Part model, mm, in its own coordinate system. Give positions to 0.01 mm unless a question says otherwise; leave off trailing zeros. Order: outer loops, then holes, each group sorted by start corner. A loop starts at its lowest first (then second) coordinate and runs counter-clockwise, first axis right, second up. Notation, with made-up numbers: M 70,58 L 123,58 A13 cw 123,66 Z; hole C 16.25,61.5 d10. An arc over 180 degrees is marked long. Answer as a JSON object with one key per item and string values.
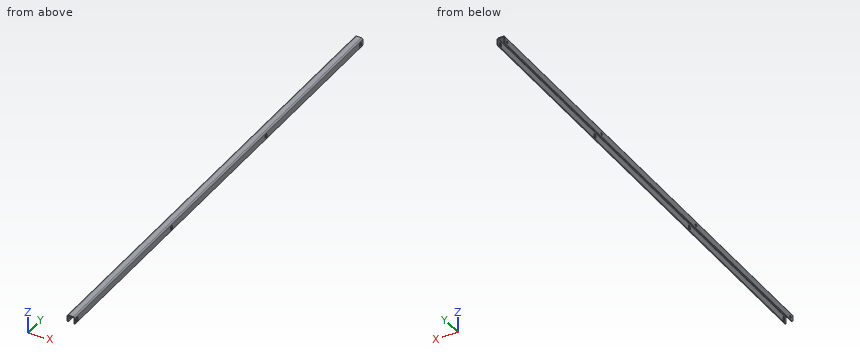
from build123d import *

# Parameters (mm, degrees)
BASE_FLANGE1_DEPTH = 1613
CUT_EXTRUDE1_REACH = 1615.344
SKETCH6_R          = 4.5
FILLET1_R          = 3
CUT_EXTRUDE2_REACH = 1615.344
LPATTERN1_COUNT    = 4
LPATTERN1_PITCH    = 529


# Sheet-metal steps are written as plain solids
with BuildPart() as part:
    # Sketch1 → Base-Flange1 (new body)
    with BuildSketch(Plane(origin=(0, 0, 0), x_dir=(1, 0, 0), z_dir=(0, 1, 0))):
        with BuildLine():
            Line((-12.5, 25), (-12.5, 4.5))
            ThreePointArc((-12.5, 4.5), (-11.181980515, 1.318019485), (-8, 0))
            Line((-8, 0), (8, 0))
            ThreePointArc((8, 0), (11.181980515, 1.318019485), (12.5, 4.5))
            Line((12.5, 4.5), (12.5, 25))
            Line((12.5, 25), (9.5, 25))
            Line((9.5, 25), (9.5, 4.5))
            ThreePointArc((9.5, 4.5), (9.060660172, 3.439339828), (8, 3))
            Line((8, 3), (-8, 3))
            ThreePointArc((-8, 3), (-9.060660172, 3.439339828), (-9.5, 4.5))
            Line((-9.5, 4.5), (-9.5, 25))
            Line((-9.5, 25), (-12.5, 25))
        make_face()
    extrude(amount=BASE_FLANGE1_DEPTH)

    # Sketch6 → Cut-Extrude1 (cut, up to next)
    with BuildSketch(Plane(origin=(-9.5, 0, 0), x_dir=(0, 0, -1), z_dir=(1, 0, 0)), mode=Mode.PRIVATE) as cut_extrude1_sk1:
        with Locations((15.5, 13)):
            Circle(SKETCH6_R)
    cut_extrude1_tool1 = extrude(cut_extrude1_sk1.sketch, amount=-CUT_EXTRUDE1_REACH, mode=Mode.PRIVATE) & part.part
    cut_extrude1 = cut_extrude1_tool1.solids().sort_by_distance((-9.5, 13, -15.5))[0]
    add(cut_extrude1, mode=Mode.SUBTRACT)

    # Fillet1
    fillet1_edges = [part.edges().sort_by_distance(p)[0] for p in [
        (11, 0, -25),
        (-11, 0, -25),
        (11, 1613, -25),
        (-11, 1613, -25),
    ]]
    fillet(fillet1_edges, radius=FILLET1_R)

    # Sketch7 → Cut-Extrude2 (cut, up to next)
    with BuildSketch(Plane.ZY.offset(-9.5), mode=Mode.PRIVATE) as cut_extrude2_sk1:
        with BuildLine():
            Line((-18.5, 18), (-12.5, 18))
            ThreePointArc((-12.5, 18), (-7.5, 13), (-12.5, 8))
            Line((-12.5, 8), (-18.5, 8))
            ThreePointArc((-18.5, 8), (-23.5, 13), (-18.5, 18))
        make_face()
    cut_extrude2_tool1 = extrude(cut_extrude2_sk1.sketch, amount=-CUT_EXTRUDE2_REACH, mode=Mode.PRIVATE) & part.part
    cut_extrude2 = cut_extrude2_tool1.solids().sort_by_distance((9.5, 13, -15.5))[0]
    add(cut_extrude2, mode=Mode.SUBTRACT)

    # LPattern1: Cut-Extrude1, Cut-Extrude2 ×4
    with Locations(*[(0, i * LPATTERN1_PITCH, 0) for i in range(1, LPATTERN1_COUNT)]):
        add(cut_extrude1, mode=Mode.SUBTRACT)
        add(cut_extrude2, mode=Mode.SUBTRACT)


solid = part.part
1. Pin check, flat tips, straight feed: P1, Ø5, axis at x = 6.5, z = -15.5, coming from the +Y side; P2, Ø13, axis at x = 2, y = 529, coming from the -Z side. Stop position of each tip, or through.
Worked answers:
{"P1": "passes through", "P2": "stops at z = -3.09"}
2. Probe line 1 along Y through (x, z) = (-10.25, -15.5); line 2 along X through (y, z) = (1268.5, -6.25); line 3 along Y through (x, z) = (-10.75, -13). List the from-to ranges inside material, lowest first.
Worked answers:
{"line 1": "y = 0 to 8.5, 17.5 to 537.5, 546.5 to 1066.5, 1075.5 to 1595.5, 1604.5 to 1613", "line 2": "x = -12.5 to -9.5, 9.5 to 12.5", "line 3": "y = 0 to 9.26, 16.74 to 538.26, 545.74 to 1067.26, 1074.74 to 1596.26, 1603.74 to 1613"}
3. Cut at B-B on x = -2. Give the cut face in (y, z).
Worked answers:
{"outline": "M 0,-3 L 1613,-3 L 1613,0 L 0,0 Z"}
4. Cut at A-A on y = 350.5. Give the cut face in (x, z), plus the area to 3 significant figures.
Worked answers:
{"outline": "M -12.5,-25 L -9.5,-25 L -9.5,-4.5 A1.5 cw -8,-3 L 8,-3 A1.5 cw 9.5,-4.5 L 9.5,-25 L 12.5,-25 L 12.5,-4.5 A4.5 ccw 8,0 L -8,0 A4.5 ccw -12.5,-4.5 Z", "area": "199 mm^2"}
